The figure shows three views and two pictorial views of one solid part (mm, origin at its lowest corner). Answer the questions. A direction names the side the tool comes from. Give positions to 0.01 mm unless a question says otherwise; leave off trailing zeros. Write each loop counter-clockwise with the first axis right and the second up, starting at its lowest first coordinate (ties: lowest second). Pieces come first, ordered by that corner, then holes. Notation, with made-up numbers: (-30, -32.75) -> (20, -32.75) arc R19 ccw to (20, -17.75) -> close; hole circle Ø10 at (-26, 51). An arc over 180 degrees is marked (long way). Use a Markdown table: item, result.
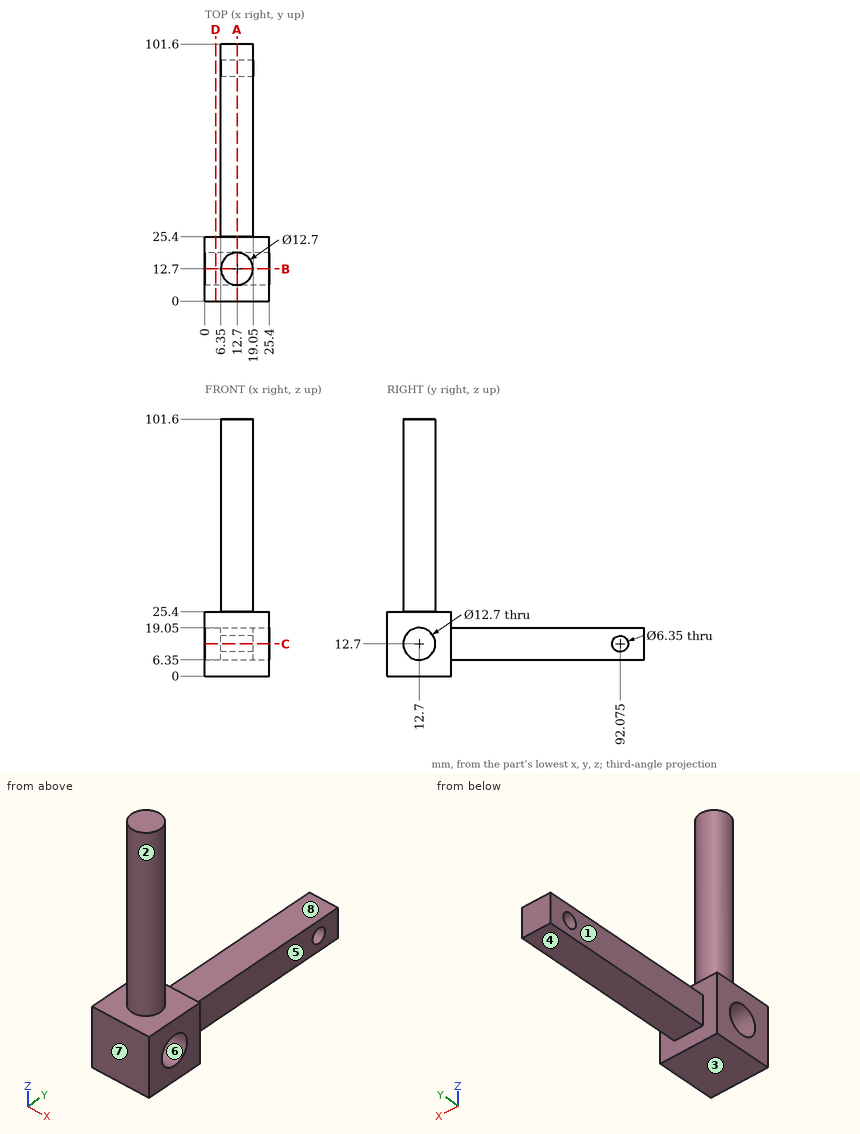
Item 1: For a pull along Z with two mould halves and no side action, classify the marked faces 6, 7 and 8 as +Z half, -Z half, draft (parallel to the pull), parting line (faces both ways), or undercut.
Return value:
| item | result |
|---|---|
| face 6 | undercut |
| face 7 | draft |
| face 8 | +Z half |
Item 2: Straight lines are drawn through the part: line 1 along Z through (x, y) = (8, 12.7); line 2 along Y through (x, z) = (9.5, 10.5); line 3 along Z through (x, y) = (14.5, 93.5). For each, find the intervals that lie inside material, in ascending order. Write a range as [from, to].
Return value:
| item | result |
|---|---|
| line 1 | [0, 6.35], [19.05, 101.6] |
| line 2 | [0, 6.74], [18.66, 89.79], [94.36, 101.6] |
| line 3 | [6.35, 9.86], [15.54, 19.05] |
Item 3: A cutting plane is placed at A-A (x = 12.7). Give the vertices of the cut face in (y, z) (3 decimals).
Return value:
| item | result |
|---|---|
| outline | (0, 0) -> (25.4, 0) -> (25.4, 6.35) -> (101.6, 6.35) -> (101.6, 19.05) -> (25.4, 19.05) -> (25.4, 25.4) -> (19.05, 25.4) -> (19.05, 101.6) -> (6.35, 101.6) -> (6.35, 25.4) -> (0, 25.4) -> close; hole circle Ø12.7 at (12.7, 12.7); hole circle Ø6.35 at (92.075, 12.7) |
Item 4: A cutting plane is placed at B-B (y = 12.7). Give the vertices of the cut face in (x, z), then the cut area to 3 significant figures.
Return value:
| item | result |
|---|---|
| outline | (0, 0) -> (25.4, 0) -> (25.4, 6.35) -> (0, 6.35) -> close; (0, 19.05) -> (25.4, 19.05) -> (25.4, 25.4) -> (19.05, 25.4) -> (19.05, 101.6) -> (6.35, 101.6) -> (6.35, 25.4) -> (0, 25.4) -> close |
| area | 1,290 mm^2 |
Item 5: A tool of negligible diameter and unlimited length cuts with its end or side. For the marked faces 1, 2, 3, 4 and 5, from which of +Z, -Z, +X, -X, +Y, -Y can it reach the whole face along a straight path? Write none if from no direction.
Return value:
| item | result |
|---|---|
| face 1 | +Z, -Z, -X, +Y |
| face 2 | +Z |
| face 3 | -Z, +X, -X, +Y, -Y |
| face 4 | -Z, +X, -X, +Y |
| face 5 | +Z, -Z, +X, +Y |
Item 6: A cutting plane is placed at D-D (x = 4.25). Give the vertices of the cut face in (y, z), then the cut area to 3 significant figures.
Return value:
| item | result |
|---|---|
| outline | (0, 0) -> (25.4, 0) -> (25.4, 25.4) -> (0, 25.4) -> close; hole circle Ø12.7 at (12.7, 12.7) |
| area | 518 mm^2 |
Item 7: Each of these flat-tipped pins is pushed along its axis until it touches: P1, Ø8, axis at y = 17, z = 86.5, coming from the +X side; P2, Ø10, axis at x = 13.5, y = 61, coming from the +Z side; P3, Ø3, axis at x = 11, z = 66, coming from the +Y side. Where does it stop, or does it pass through?
Return value:
| item | result |
|---|---|
| P1 | x = 19.04 |
| P2 | z = 19.05 |
| P3 | y = 19.05 |
Item 8: A cutting plane is placed at C-C (z = 12.7). Give the vertices of the cut face in (x, y), then the cut area to 3 significant figures.
Return value:
| item | result |
|---|---|
| outline | (0, 0) -> (25.4, 0) -> (25.4, 6.35) -> (0, 6.35) -> close; (0, 19.05) -> (25.4, 19.05) -> (25.4, 25.4) -> (19.05, 25.4) -> (19.05, 88.9) -> (6.35, 88.9) -> (6.35, 25.4) -> (0, 25.4) -> close; (6.35, 95.25) -> (19.05, 95.25) -> (19.05, 101.6) -> (6.35, 101.6) -> close |
| area | 1,210 mm^2 |
